Autodesk Inventor part; units mm, degrees
ref_plane "YZ Plane" through (0, 0, 0) normal (1, 0, 0) x (0, 1, 0)
ref_plane "XZ Plane" through (0, 0, 0) normal (0, 1, 0) x (-1, 0, 0)
ref_plane "XY Plane" through (0, 0, 0) normal (0, 0, 1) x (1, 0, 0)
sketch "Sketch1" plane through (0, 0, 0) normal (1, 0, 0) x (0, 1, 0)
  line L0 (0, 0) -> (25.4, 0)
  line L1 (25.4, 0) -> (25.4, 3.175)
  line L2 (25.4, 3.175) -> (0, 3.175)
  line L3 (0, 3.175) -> (0, 0)
  line L4 (0, 0) -> (0, 25.4)
  line L5 (0, 25.4) -> (3.175, 25.4)
  line L6 (3.175, 25.4) -> (3.175, 3.175)
  point P0 (3.175, 3.175)
  dimension "d0" = 25.4
  dimension "d1" = 3.175
  dimension "d2" = 25.4
  dimension "d3" = 25.4
  dimension "d4" = 3.175
  dimension "d5" = 90
extrude "Extrusion1" add sketch "Sketch1" along normal blind 150
properties part number "SOPORTE LATERAL DE GUIA CILINDRICA"
Input: part model. Units: mm. Frame: model coordinates. A direction names the side the tool comes from. Give positions to 0.01 mm unless a question says otherwise; leave off trailing zeros. Order: outer loops, then holes, each group sorted by start corner. A loop starts at its lowest first (then second) coordinate and runs counter-clockwise, first axis right, second up. Notation, with made-up numbers: M 47.25,33.5 L 101.25,33.5 A10 cw 101.25,40.5 Z; hole C 37,-25 d11. An arc over 180 degrees is marked long. One line per question, with ' | ' between items. Start each with the question number.
1. Access query for faces 1 (the face through (74, 2, 25.4)), 2 (the face through (74, 14, 3.175)). Directions: +Z, -Z, +X, -X, +Y, -Y. A direction counts if a zero-diameter tool reaches every point of the face in a straight line with its end or side. Return the directions, or none.
2. First-contact query: pin 1 Ø1 at (x, z) = (90, 12) entering from +Y (3 decimals); pin 2 Ø1.5 at (x, y) = (35, 9) entering from +Z (3 decimals). Flat tips, straight axial feed; report the tip coordinate or a pass-through.
3. Section query B-B (z = 10.75). Return the cut outline in (x, y) (3 decimals), and give its area (3 significant figures).
4. Material intervals for probe 1 along Z at (x, y) = (123, 17) (3 decimals), sorted ascending. Write a range as [from, to].
5. Section query A-A (x = 133.5). Return the cut outline in (y, z) (3 decimals).
Here are the results:
1) face 1: +Z, +X, -X, +Y, -Y | face 2: +Z, +X, -X, +Y
2) pin 1: y = 3.175 | pin 2: z = 3.175
3) outline: M 0,0 L 150,0 L 150,3.175 L 0,3.175 Z | area: 476 mm²
4) probe 1: [0, 3.175]
5) outline: M 0,0 L 25.4,0 L 25.4,3.175 L 3.175,3.175 L 3.175,25.4 L 0,25.4 Z
